Could you check a few things on this drawing? It's one solid part, dimensions in mm from its lowest x, y, z. A direction names the side the tool comes from. Coordinates: 2 decimals unless noted, no trailing zeros. Order: outer loops, then holes, each group sorted by start corner. A loop starts at its lowest first (then second) coordinate and runs counter-clockwise, first axis right, second up. Notation, with made-up numbers: (-0.5, 88.5) -> (54.5, 88.5) arc R21 ccw to (54.5, 118.5) -> close; hole circle Ø1 at (72, 37.25). An arc over 180 degrees is marked (long way). Use a Markdown table: item, result. Add a question column.
1. Suppose I cut it at D-D, the plane y = 14.5. List the corners of the cut face in (x, z) for me.
2. For the marked faces 4, 5 and 6, which set-ups out of +Z, -Z, +X, -X, +Y, -Y let a thin tool reach every point of the face, with its end or its side?
3. If I drill on line 1 along Y through (x, z) = (12, 1.1); line 2 along Y through (x, z) = (13.75, 1.7) (1 decimal); line 3 along Y through (x, z) = (13.25, 1.75) (1 decimal), over which ranges is the centre line in solid material (lowest first)? Write a range as from..to.
4. For pin 1 Ø1.1 at (x, z) = (23, 1) entering from +Y; pin 2 Ø2 at (x, y) = (9, 24) entering from +Z, each with a flat end and sliding along its axis, tell me the tip position at first contact or that it passes through.
5. Suppose I cut it at A-A, the plane x = 12. List the corners of the cut face in (y, z) for me, then the cut area to 3 significant figures.
6. Suppose I cut it at C-C, the plane z = 1.6. State how many separate pieces and enclosed holes the cut face has, then the cut area to 3 significant figures.
7. Suppose I cut it at B-B, the plane y = 24.5. List the corners of the cut face in (x, z) for me.
8. We'd pull the mould along X, two halves only. Please class the marked faces 1, 2 and 3: pulls with the +X half, pulls with the -X half, needs draft (parallel to the pull), parting line crosses it, or undercut.
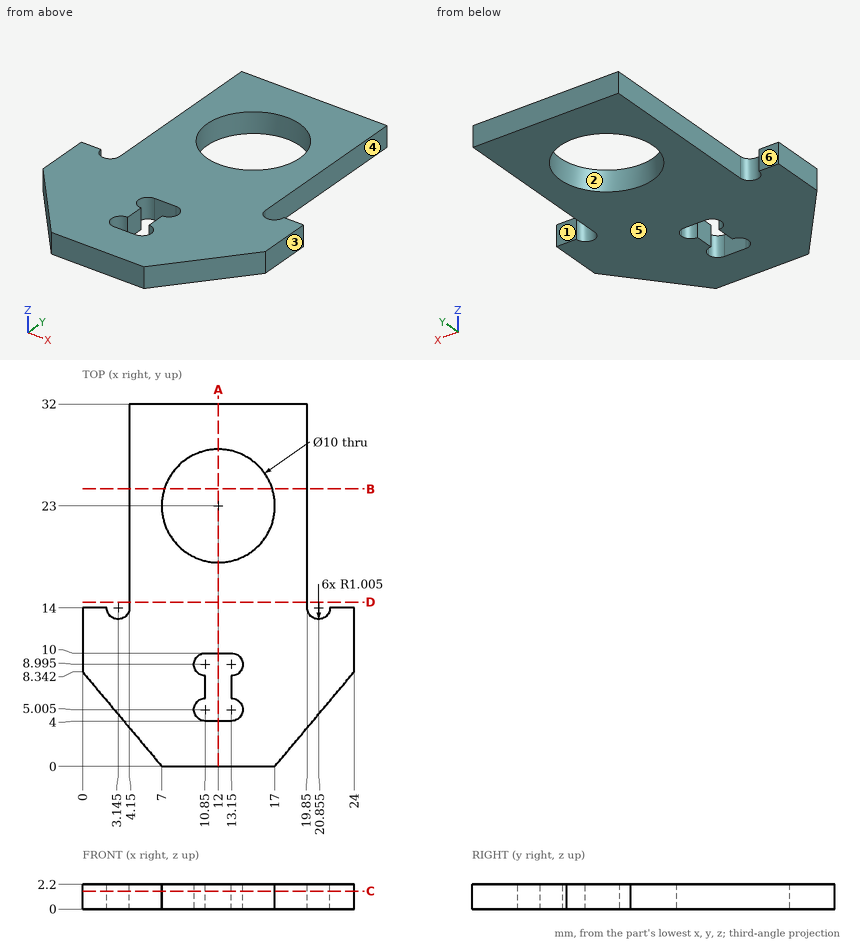
Worked out:
| question | item | result |
|---|---|---|
| 1 | outline | (4.15, 0) -> (19.85, 0) -> (19.85, 2.2) -> (4.15, 2.2) -> close |
| 2 | face 4 | +Z, -Z, +X, +Y |
| 2 | face 5 | -Z, +X, -X, +Y, -Y |
| 2 | face 6 | +Z, -Z, -X, +Y |
| 3 | line 1 | y = 0..4, 10..18, 28..32 |
| 3 | line 2 | y = 0..4.2, 5.8..8.2, 9.8..18.3, 27.7..32 |
| 3 | line 3 | y = 0..4, 6..8, 10..18.2, 27.8..32 |
| 4 | pin 1 | stops at y = 14 |
| 4 | pin 2 | passes through |
| 5 | outline | (0, 0) -> (4, 0) -> (4, 2.2) -> (0, 2.2) -> close; (10, 0) -> (18, 0) -> (18, 2.2) -> (10, 2.2) -> close; (28, 0) -> (32, 0) -> (32, 2.2) -> (28, 2.2) -> close |
| 5 | area | 35.2 mm² |
| 6 | separate pieces | 1 |
| 6 | enclosed holes | 2 |
| 6 | area | 458 mm² |
| 7 | outline | (4.15, 0) -> (7.23, 0) -> (7.23, 2.2) -> (4.15, 2.2) -> close; (16.77, 0) -> (19.85, 0) -> (19.85, 2.2) -> (16.77, 2.2) -> close |
| 8 | face 1 | needs draft |
| 8 | face 2 | undercut |
| 8 | face 3 | pulls with the +X half |
